from build123d import *

# Parameters (mm, degrees)
SKETCH_1_W      = 40
SKETCH_1_H      = 30
SKETCH_1_R      = 2.1
SKETCH_1_W_2    = 3
SKETCH_1_H_2    = 20
EXTRUDE_1_DEPTH = 3


with BuildPart() as part:
    # 草图1 → 凸台-拉伸1 (new body)
    with BuildSketch(Plane(origin=(0, 0, 0), x_dir=(1, 0, 0), z_dir=(0, 1, 0))):
        with Locations((20, -15)):
            Rectangle(SKETCH_1_W, SKETCH_1_H)
        with Locations(Location((20, -23, 0), (0, 0, 270))):
            Circle(SKETCH_1_R, mode=Mode.SUBTRACT)
        with Locations(Location((20, -7, 0), (0, 0, 270))):
            Circle(SKETCH_1_R, mode=Mode.SUBTRACT)
        with Locations((6, -15)):
            Rectangle(SKETCH_1_W_2, SKETCH_1_H_2, mode=Mode.SUBTRACT)
        with Locations((34, -15)):
            Rectangle(SKETCH_1_W_2, SKETCH_1_H_2, mode=Mode.SUBTRACT)
        with Locations((27.5, -15)):
            Rectangle(SKETCH_1_W_2, SKETCH_1_H_2, mode=Mode.SUBTRACT)
        with Locations((12.5, -15)):
            Rectangle(SKETCH_1_W_2, SKETCH_1_H_2, mode=Mode.SUBTRACT)
    extrude(amount=EXTRUDE_1_DEPTH)


solid = part.part
For this review, take the finished solid that the model builds, in its own axes (mm). A direction names the side the tool comes from. Round coordinates to 2 decimals unless told otherwise and drop trailing zeros. Order: outer loops, then holes, each group sorted by start corner. A loop starts at its lowest first (then second) coordinate and runs counter-clockwise, first axis right, second up. Notation, with made-up numbers: M -18,-21 L 17,-21 A30 cw 17,13 Z; hole C 2.25,16 d6. An arc over 180 degrees is marked long. Use a Markdown table: item, result. Add a question column.
Item 1: Add section D-D, the plane z = 7. Give the boundary of the cut face in (x, y).
Item 2: To check wall thickness, follow line 1 along X through (y, z) = (1.75, 23); line 2 along X through (y, z) = (1.9, 12); line 3 along Z through (x, y) = (5.5, 0.4). State the ranges of each line that lie inside material, in increasing order.
Item 3: Add section B-B, the plane y = 1.7. Give the boundary of the cut face in (x, z), then the cut area to 3 significant figures.
Item 4: Add section A-A, the plane x = 20. Give the boundary of the cut face in (y, z), then the cut area to 3 significant figures.
Item 5: Mouldability with a two-part tool opening along Z and no side actions: class faces 3 (the flat face through (20, 1, 0)), 4 (the flat face through (20, 1, 30)), 5 (the flat face through (12, 1, 5)), 6 (the flat face through (34, 1, 5)) as released by +Z, released by -Z, zero draft, split by the parting line, or undercut.
Item 6: Tool access review of faces 1 (the flat face through (27, 1, 5)), 2 (the flat face through (0, 1, 15)): name each direction out of +Z, -Z, +X, -X, +Y, -Y from which nothing blocks a thin tool from reaching the whole face with its end or side.
Item 7: Add section C-C, the plane x = 35. Give the boundary of the cut face in (y, z), then the cut area to 3 significant figures.
Item 8: Insertion check: pin 1 (5 mm diameter, centred on x = 13.5, z = 11.5, fed in from +Y); pin 2 (2.5 mm diameter, centred on x = 20, z = 7, fed in from -Y). Each pin has a flat end and moves straight along its axis. Give the tip position at first contact, or say it passes through.
Geometry results:
| question | item | result |
|---|---|---|
| 1 | outline | M 0,0 L 4.5,0 L 4.5,3 L 0,3 Z; M 7.5,0 L 11,0 L 11,3 L 7.5,3 Z; M 14,0 L 17.9,0 L 17.9,3 L 14,3 Z; M 22.1,0 L 26,0 L 26,3 L 22.1,3 Z; M 29,0 L 32.5,0 L 32.5,3 L 29,3 Z; M 35.5,0 L 40,0 L 40,3 L 35.5,3 Z |
| 2 | line 1 | x = 0 to 4.5, 7.5 to 11, 14 to 17.9, 22.1 to 26, 29 to 32.5, 35.5 to 40 |
| 2 | line 2 | x = 0 to 4.5, 7.5 to 11, 14 to 26, 29 to 32.5, 35.5 to 40 |
| 2 | line 3 | z = 0 to 5, 25 to 30 |
| 3 | outline | M 0,0 L 40,0 L 40,30 L 0,30 Z; hole M 4.5,5 L 7.5,5 L 7.5,25 L 4.5,25 Z; hole M 11,5 L 14,5 L 14,25 L 11,25 Z; hole C 20,7 d4.2; hole C 20,23 d4.2; hole M 26,5 L 29,5 L 29,25 L 26,25 Z; hole M 32.5,5 L 35.5,5 L 35.5,25 L 32.5,25 Z |
| 3 | area | 932 mm² |
| 4 | outline | M 0,0 L 3,0 L 3,4.9 L 0,4.9 Z; M 0,9.1 L 3,9.1 L 3,20.9 L 0,20.9 Z; M 0,25.1 L 3,25.1 L 3,30 L 0,30 Z |
| 4 | area | 64.8 mm² |
| 5 | face 3 | released by -Z |
| 5 | face 4 | released by +Z |
| 5 | face 5 | undercut |
| 5 | face 6 | undercut |
| 6 | face 1 | +Y, -Y |
| 6 | face 2 | +Z, -Z, -X, +Y, -Y |
| 7 | outline | M 0,0 L 3,0 L 3,5 L 0,5 Z; M 0,25 L 3,25 L 3,30 L 0,30 Z |
| 7 | area | 30.0 mm² |
| 8 | pin 1 | stops at y = 3 |
| 8 | pin 2 | passes through |
